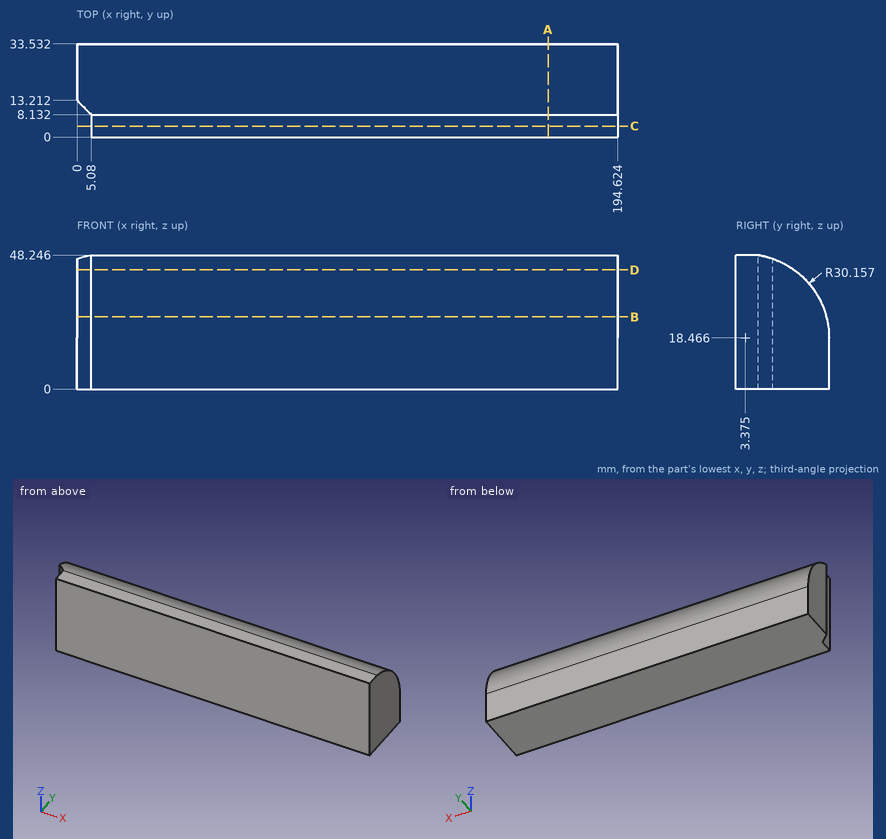
Geometry check sheet. Reference: drawing and pictorial views, mm from the part's lowest x, y, z. Round coordinates to 2 decimals unless told otherwise and drop trailing zeros. Loops run counter-clockwise (first coordinate to the right, second up) from the corner with the lowest first, then second, coordinate; pieces in that order, holes last. Notation, with made-up numbers: (88, 43.25) -> (123, 43.25) arc R21 ccw to (123, 52.25) -> close; hole circle Ø6 at (-3.5, -7.75). An arc over 180 degrees is marked (long way). Answer as a JSON object with one key per item and string values. Group by question number.
Item 1: Cross-section at B-B, the plane z = 26. Record the cut outline in (x, y), plus the area to 3 significant figures.
Item 2: Cross-section at A-A, the plane x = 169.5. Record the cut outline in (y, z) (1 decimal), plus the area to 3 significant figures.
Item 3: Cross-section at C-C, the plane y = 4. Record the cut outline in (x, z).
Item 4: Thickness scan on line 1 along X through (y, z) = (3, 42.5); line 2 along Y through (x, z) = (114.5, 19.5); line 3 along Z through (x, y) = (78, 8.5) (1 decimal). Record the ranges inside material, lowest first.
Item 5: Depth check by flat-ended pin: pin 1 Ø5 at (x, z) = (105.5, 28.5) entering from +Y; pin 2 Ø4 at (y, z) = (5.5, 35) entering from -X; pin 3 Ø4 at (y, z) = (10.5, 18) entering from -X. Enter the tip coordinate at first touch or a pass-through.
Item 6: Cross-section at D-D, the plane z = 43. Record the cut outline in (x, y).
Determined:
{
 "1": {"outline": "(0, 13.21) -> (5.08, 8.13) -> (5.08, 0) -> (194.62, 0) -> (194.62, 32.58) -> (0, 32.58) -> close", "area": "6,290 mm²"},
 "2": {"outline": "(0, 0) -> (33.5, 0) -> (33.5, 18.5) arc R30.2 ccw to (8.1, 48.2) -> (0, 48.2) -> close", "area": "1,430 mm²"},
 "3": {"outline": "(5.08, 0) -> (194.62, 0) -> (194.62, 48.25) -> (5.08, 48.25) -> close"},
 "4": {"line 1": "x = 5.08 to 194.62", "line 2": "y = 0 to 33.51", "line 3": "z = 0 to 48.2"},
 "5": {"pin 1": "stops at y = 32.58", "pin 2": "stops at x = 5.08", "pin 3": "stops at x = 0.71"},
 "6": {"outline": "(0, 13.21) -> (5.08, 8.13) -> (5.08, 0) -> (194.62, 0) -> (194.62, 20.91) -> (0, 20.91) -> close"}
}
